```python
from build123d import *

# Parameters (mm, degrees)
SKETCH1_W                                           = 80
SKETCH1_H                                           = 120
BOSS_EXTRUDE1_DEPTH                                 = 5
M5_TAPPED_HOLE1_D                                   = 4.2
M5_TAPPED_HOLE1_DEPTH                               = 20
M5_TAPPED_HOLE1_TIP                                 = 1.2618073
SKETCH6_W                                           = 40
SKETCH6_H                                           = 30
CUT_EXTRUDE2_DEPTH                                  = 3
CBORE_FOR_M4_HEX_SOCKET_HEAD_CAP_SCREW1_D           = 4.5
CBORE_FOR_M4_HEX_SOCKET_HEAD_CAP_SCREW1_DEPTH       = 20
CBORE_FOR_M4_HEX_SOCKET_HEAD_CAP_SCREW1_CBORE_D     = 8
CBORE_FOR_M4_HEX_SOCKET_HEAD_CAP_SCREW1_CBORE_DEPTH = 4.4
CBORE_FOR_M4_HEX_SOCKET_HEAD_CAP_SCREW1_TIP         = 1.351936393


with BuildPart() as part:
    # Sketch1 → Boss-Extrude1 (new, symmetric)
    with BuildSketch(Plane(origin=(0, 0, 0), x_dir=(1, 0, 0), z_dir=(0, 1, 0))):
        Rectangle(SKETCH1_W, SKETCH1_H)
    extrude(amount=BOSS_EXTRUDE1_DEPTH, both=True)

    # M5 Tapped Hole1
    with Locations(Plane(origin=(40, 0, 17.5), x_dir=(0, 0, 1), z_dir=(1, 0, 0))):
        with Locations((-70.5, -0.150021458), (-35, -0.150021458), (-20, -0.150021458), (-5, -0.150021458), (35.5, -0.150021458)):
            Hole(M5_TAPPED_HOLE1_D / 2, depth=M5_TAPPED_HOLE1_DEPTH)
            with Locations((0, 0, -(M5_TAPPED_HOLE1_DEPTH + M5_TAPPED_HOLE1_TIP / 2))):  # 118° drill point
                Cone(0, M5_TAPPED_HOLE1_D / 2, M5_TAPPED_HOLE1_TIP, mode=Mode.SUBTRACT)

    # Sketch6 → Cut-Extrude2 (cut)
    with BuildSketch(Plane.XZ.offset(5)):
        with Locations((-4.85, 0)):
            Rectangle(SKETCH6_W, SKETCH6_H)
    extrude(amount=-CUT_EXTRUDE2_DEPTH, mode=Mode.SUBTRACT)

    # CBORE for M4 Hex Socket Head Cap Screw1
    with Locations(Plane(origin=(0, 5, 0), x_dir=(1, 0, 0), z_dir=(0, 1, 0))):
        with Locations((-19.85000137, 7.5), (10.14999863, 7.5), (10.14999863, -7.5), (-19.85000137, -7.5)):
            CounterBoreHole(CBORE_FOR_M4_HEX_SOCKET_HEAD_CAP_SCREW1_D / 2, CBORE_FOR_M4_HEX_SOCKET_HEAD_CAP_SCREW1_CBORE_D / 2, CBORE_FOR_M4_HEX_SOCKET_HEAD_CAP_SCREW1_CBORE_DEPTH, depth=CBORE_FOR_M4_HEX_SOCKET_HEAD_CAP_SCREW1_DEPTH)
            with Locations((0, 0, -(CBORE_FOR_M4_HEX_SOCKET_HEAD_CAP_SCREW1_DEPTH + CBORE_FOR_M4_HEX_SOCKET_HEAD_CAP_SCREW1_TIP / 2))):  # 118° drill point
                Cone(0, CBORE_FOR_M4_HEX_SOCKET_HEAD_CAP_SCREW1_D / 2, CBORE_FOR_M4_HEX_SOCKET_HEAD_CAP_SCREW1_TIP, mode=Mode.SUBTRACT)


solid = part.part
```
Geometry: final body of the model. Coordinates: model frame, mm. A direction names the side the tool comes from. Give positions to 0.01 mm unless a question says otherwise; leave off trailing zeros. Order: outer loops, then holes, each group sorted by start corner. A loop starts at its lowest first (then second) coordinate and runs counter-clockwise, first axis right, second up. Notation, with made-up numbers: M -22,18 L -6,18 A4 cw -6,25 Z; hole C 81,-9 d9. An arc over 180 degrees is marked long. Answer as CSV lines item,"result". Start each with the question number.
1) Cut plane C-C (x = 33). Output: boundary loops of the cut face in (y, z).
2) Cut plane B-B (x = -12.5). Output: boundary loops of the cut face in (y, z).
3) Mould query, pull axis Z, two halves, no side actions, for faces 5 (the flat face through (17, -5, -1)), 6 (the flat face through (15.15, -4, 0)), 7 (the flat face through (-1, 0, -60)). Classes: +Z half, -Z half, draft (parallel to the pull), parting line (faces both ways), or undercut.
4) First-contact query: P1, Ø6, axis at x = -19.85, z = 7.5, coming from the -Y side; P2, Ø2.5, axis at x = 9.5, z = -6, coming from the +Y side; P3, Ø2.5, axis at x = -19.85, z = -7.5, coming from the +Y side. Flat tips, straight axial feed; report the tip coordinate or a pass-through.
5) Cut plane A-A (z = -7.5). Output: boundary loops of the cut face in (x, y), then the cut area to 3 significant figures.
6) Set-up query: faces 1 (the flat face through (-5, -4, 15)), 2 (the flat face through (11.9, 0.6, -5.8)), 3 (the cylindrical face through (29.9, 0.1, 14.6)), 4 (the cylindrical face through (-18.19, -0.72, -9.02)). Return all of +Z, -Z, +X, -X, +Y, -Y with unobstructed straight access to the full face (end or side cutting, diameter ignored); none if empty.
7) Line query: line 1 (Z direction, x = 7, y = -4); line 2 (Z direction, x = 30, y = -0.25); line 3 (X direction, y = 2.25, z = -11). Output: solid intervals per line, ascending. Write a range as from..to.
Findings below:
1,outline,"M -5,-60 L 5,-60 L 5,60 L -5,60 Z; hole C 0.15,-53 d4.2; hole C 0.15,-17.5 d4.2; hole C 0.15,-2.5 d4.2; hole C 0.15,12.5 d4.2; hole C 0.15,53 d4.2"
2,outline,"M -5,-60 L 5,-60 L 5,60 L -5,60 L -5,15 L -2,15 L -2,-15 L -5,-15 Z"
3,face 5,"draft"
3,face 6,"undercut"
3,face 7,"-Z half"
4,P1,"stops at y = -2"
4,P2,"stops at y = 0.6"
4,P3,"passes through"
5,outline,"M -40,-5 L -24.85,-5 L -24.85,-2 L -22.1,-2 L -22.1,0.6 L -23.85,0.6 L -23.85,5 L -40,5 Z; M -17.6,-2 L 7.9,-2 L 7.9,0.6 L 6.15,0.6 L 6.15,5 L -15.85,5 L -15.85,0.6 L -17.6,0.6 Z; M 12.4,-2 L 15.15,-2 L 15.15,-5 L 40,-5 L 40,5 L 14.15,5 L 14.15,0.6 L 12.4,0.6 Z"
5,area,"586 mm²"
6,face 1,"-Y"
6,face 2,"+Y"
6,face 3,"+X"
6,face 4,"+Y, -Y"
7,line 1,"z = -60..-15, 15..60"
7,line 2,"z = -60..-55.06, -50.94..-19.56, -15.44..-4.56, -0.44..10.44, 14.56..50.94, 55.06..60"
7,line 3,"x = -40..-21.79, -17.91..8.21, 12.09..40"
